Part print with two shaded views. Sizes in mm from the minimum x, y, z corner. A direction names the side the tool comes from. Coordinates: 2 decimals unless noted, no trailing zeros. Loops run counter-clockwise (first coordinate to the right, second up) from the corner with the lowest first, then second, coordinate; pieces in that order, holes last. Notation, with made-up numbers: M -9,19 L 10,19 A26 ccw 10,53 Z; hole C 28.5,-4 d10. An arc over 180 degrees is marked long. Use CSV: the item, a comma, the result in double quotes. Start each with the question number.
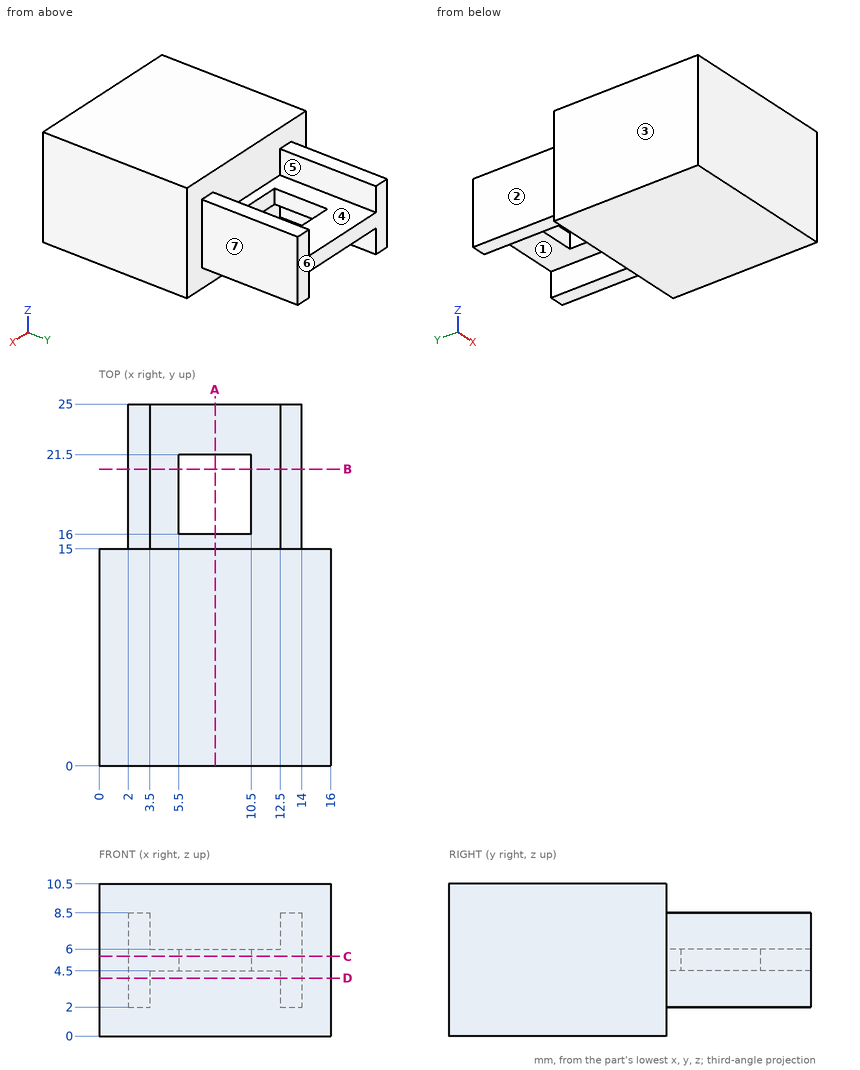
1. Two-plate mould, pull along X, no slides. Class the marked faces 5, 6 and 7: pulls with the +X half, pulls with the -X half, needs draft (parallel to the pull), parting line crosses it, or undercut.
2. Slice it at A-A, the plane x = 8. List the corners of the cut face in (y, z).
3. Slice it at C-C, the plane z = 5.5. List the corners of the cut face in (x, y).
4. Pin check, flat tips, straight feed: pin 1 (2 mm diameter, centred on y = 19.5, z = 6.5, fed in from +X); pin 2 (1.5 mm diameter, centred on x = 6.5, z = 3.5, fed in from +Y); pin 3 (0.8 mm diameter, centred on x = 2.5, y = 20.5, fed in from -Z). Stop position of each tip, or through.
5. Slice it at D-D, the plane z = 4. List the corners of the cut face in (x, y).
6. Slice it at B-B, the plane y = 20.5. List the corners of the cut face in (x, z), and give its area (3 significant figures).
7. Tool access for the marked faces 1, 2, 3 and 4: list every direction of +Z, -Z, +X, -X, +Y, -Y with a clear straight run to the whole face (end or side of a thin tool).
8. Wall check: probe 1 along X at (y, z) = (19.75, 2.5); probe 2 along Y at (x, z) = (6.75, 5.75); probe 3 along Z at (x, y) = (3, 16.5). Give the ranges that are in metal, low to high.
Found:
1,face 5,"undercut"
1,face 6,"needs draft"
1,face 7,"pulls with the +X half"
2,outline,"M 0,0 L 15,0 L 15,4.5 L 16,4.5 L 16,6 L 15,6 L 15,10.5 L 0,10.5 Z; M 21.5,4.5 L 25,4.5 L 25,6 L 21.5,6 Z"
3,outline,"M 0,0 L 16,0 L 16,15 L 14,15 L 14,25 L 2,25 L 2,15 L 0,15 Z; hole M 5.5,16 L 10.5,16 L 10.5,21.5 L 5.5,21.5 Z"
4,pin 1,"x = 14"
4,pin 2,"y = 15"
4,pin 3,"z = 2"
5,outline,"M 0,0 L 16,0 L 16,15 L 14,15 L 14,25 L 12.5,25 L 12.5,15 L 3.5,15 L 3.5,25 L 2,25 L 2,15 L 0,15 Z"
6,outline,"M 2,2 L 3.5,2 L 3.5,4.5 L 5.5,4.5 L 5.5,6 L 3.5,6 L 3.5,8.5 L 2,8.5 Z; M 10.5,4.5 L 12.5,4.5 L 12.5,2 L 14,2 L 14,8.5 L 12.5,8.5 L 12.5,6 L 10.5,6 Z"
6,area,"25.5 mm^2"
7,face 1,"-Z, +Y"
7,face 2,"+Z, -Z, -X, +Y"
7,face 3,"+Z, -Z, -X, +Y, -Y"
7,face 4,"+Z, +Y"
8,probe 1,"2 to 3.5, 12.5 to 14"
8,probe 2,"0 to 16, 21.5 to 25"
8,probe 3,"2 to 8.5"
